from build123d import *

# Parameters (mm, degrees)
SCHIZZO1_W                               = 90
SCHIZZO1_H                               = 80
ESTRUSIONE_ESTRUSIONE1_DEPTH             = 10
RACCORDO1_R                              = 10
FORO_SVASATO_PER_VITE_M2_5_1_D           = 3.1
FORO_SVASATO_PER_VITE_M2_5_1_CSINK_D     = 5.5
FORO_SVASATO_PER_VITE_M2_5_1_CSINK_ANGLE = 90
SCHIZZO4_W                               = 30
SCHIZZO4_H                               = 15
ESTRUSIONE_ESTRUSIONE2_DEPTH             = 13
FORO_SVASATO_PER_VITE_M2_5_2_D           = 3.1
FORO_SVASATO_PER_VITE_M2_5_2_DEPTH       = 15
FORO_SVASATO_PER_VITE_M2_5_2_CSINK_D     = 5.5
FORO_SVASATO_PER_VITE_M2_5_2_CSINK_ANGLE = 90
FORO_SVASATO_PER_VITE_M2_5_2_TIP         = 0.931333959
RACCORDO2_R                              = 3
SCHIZZO5_R                               = 1.7
TAGLIO_ESTRUSIONE4_DEPTH                 = 15
TAGLIO_ESTRUSIONE5_START                 = -15
SCHIZZO6_R                               = 1.7
TAGLIO_ESTRUSIONE5_DEPTH                 = 15


with BuildPart() as part:
    # Schizzo1 → Estrusione-Estrusione1 (new body)
    with BuildSketch(Plane(origin=(0, 0, 0), x_dir=(1, 0, 0), z_dir=(0, 1, 0))):
        with Locations((-2.6, -4.4)):
            Rectangle(SCHIZZO1_W, SCHIZZO1_H)
    extrude(amount=ESTRUSIONE_ESTRUSIONE1_DEPTH)

    # Raccordo1
    raccordo1_edges = [part.edges().sort_by_distance(p)[0] for p in [
        (42.4, 5, -35.6),
        (42.4, 5, 44.4),
        (-47.6, 5, 44.4),
        (-47.6, 5, -35.6),
    ]]
    fillet(raccordo1_edges, radius=RACCORDO1_R)

    # Foro svasato per Vite M2.5-1 (through all)
    with Locations(Plane(origin=(12.4, 10, -15.6), x_dir=(0, 0, 1), z_dir=(0, 1, 0))):
        with Locations((0, 0), (40, 0)):
            CounterSinkHole(FORO_SVASATO_PER_VITE_M2_5_1_D / 2, FORO_SVASATO_PER_VITE_M2_5_1_CSINK_D / 2, counter_sink_angle=FORO_SVASATO_PER_VITE_M2_5_1_CSINK_ANGLE)

    # Schizzo4 → Estrusione-Estrusione2 (add)
    with BuildSketch(Plane(origin=(0, 10, 0), x_dir=(1, 0, 0), z_dir=(0, 1, 0))):
        with Locations((-17.6, 13.1)):
            Rectangle(SCHIZZO4_W, SCHIZZO4_H)
        with Locations((-17.6, -21.9)):
            Rectangle(SCHIZZO4_W, SCHIZZO4_H)
    extrude(amount=ESTRUSIONE_ESTRUSIONE2_DEPTH)

    # Foro svasato per Vite M2.5-2
    with Locations(Plane(origin=(-10.6, 14.5, 29.4), x_dir=(1, 0, 0), z_dir=(0, 0, 1))):
        with Locations((0, 0)):
            CounterSinkHole(FORO_SVASATO_PER_VITE_M2_5_2_D / 2, FORO_SVASATO_PER_VITE_M2_5_2_CSINK_D / 2, depth=FORO_SVASATO_PER_VITE_M2_5_2_DEPTH, counter_sink_angle=FORO_SVASATO_PER_VITE_M2_5_2_CSINK_ANGLE)
            with Locations((0, 0, -(FORO_SVASATO_PER_VITE_M2_5_2_DEPTH + FORO_SVASATO_PER_VITE_M2_5_2_TIP / 2))):  # 118° drill point
                Cone(0, FORO_SVASATO_PER_VITE_M2_5_2_D / 2, FORO_SVASATO_PER_VITE_M2_5_2_TIP, mode=Mode.SUBTRACT)

    # Raccordo2
    raccordo2_edges = [part.edges().sort_by_distance(p)[0] for p in [
        (-2.6, 16.5, -20.6),
        (-32.6, 16.5, -20.6),
        (-32.6, 16.5, -5.6),
        (-2.6, 16.5, -5.6),
        (-2.6, 16.5, 14.4),
        (-32.6, 16.5, 14.4),
        (-32.6, 16.5, 29.4),
        (-2.6, 16.5, 29.4),
    ]]
    fillet(raccordo2_edges, radius=RACCORDO2_R)

    # Schizzo5 → Taglio-Estrusione4 (cut)
    with BuildSketch(Plane(origin=(0, 0, -20.6), x_dir=(-1, 0, 0), z_dir=(0, 0, -1))):
        with Locations((10.6, 14.5)):
            Circle(SCHIZZO5_R)
        with Locations((24.6, 14.5)):
            Circle(SCHIZZO5_R)
    extrude(amount=-TAGLIO_ESTRUSIONE4_DEPTH, mode=Mode.SUBTRACT)

    # Schizzo6 → Taglio-Estrusione5 (cut)
    with BuildSketch(Plane.XY.offset(29.4).offset(TAGLIO_ESTRUSIONE5_START)):
        with Locations(Location((-24.6, 14.5, 0), (0, 0, 180))):
            Circle(SCHIZZO6_R)
    extrude(amount=TAGLIO_ESTRUSIONE5_DEPTH, mode=Mode.SUBTRACT)


solid = part.part
Geometry: final body of the model. Coordinates: model frame, mm. A direction names the side the tool comes from. Give positions to 0.01 mm unless a question says otherwise; leave off trailing zeros. Order: outer loops, then holes, each group sorted by start corner. A loop starts at its lowest first (then second) coordinate and runs counter-clockwise, first axis right, second up. Notation, with made-up numbers: (-18.5, 85.25) -> (34.5, 85.25) arc R18 ccw to (34.5, 108.25) -> close; hole circle Ø10 at (83.5, 24). An arc over 180 degrees is marked (long way). Answer as a JSON object with one key per item and string values.
Q1. Draft query along X for faces 5 (the cylindrical face through (-22.9, 14.43, 21.8)), 6 (the flat face through (-18, 16, -5.6)), 7 (the cylindrical face through (-3.46, 16.59, -6.5)). Return one class per face: released by +X, released by -X, zero draft, split by the parting line, or undercut.
Entries:
{"face 5": "undercut", "face 6": "zero draft", "face 7": "released by +X"}
Q2. Access query for faces 1 (the cylindrical face through (-31.74, 16.59, -19.7)), 2 (the flat face through (-2.6, 16, -13)), 3 (the flat face through (-18, 16, 29.4)), 4 (the flat face through (-18, 16, -20.6)). Directions: +Z, -Z, +X, -X, +Y, -Y. A direction counts if a zero-diameter tool reaches every point of the face in a straight line with its end or side. Return the directions, or none.
Entries:
{"face 1": "-Z, -X, +Y", "face 2": "+Z, -Z, +X, +Y", "face 3": "+Z, +X, -X, +Y", "face 4": "-Z, +X, -X, +Y"}
Q3. Material intervals for probe 1 along Y at (x, z) = (-24.6, 22); probe 2 along Z at (x, y) = (-28.5, 19); probe 3 along Z at (x, y) = (12.4, 7.25), sorted ascending.
Entries:
{"probe 1": "y = 0 to 12.8, 16.2 to 23", "probe 2": "z = -20.6 to -5.6, 14.4 to 29.4", "probe 3": "z = -35.6 to -17.15, -14.05 to 22.85, 25.95 to 44.4"}
Q4. Section D-D (y = 21.5). Output: boundary loops of the cut face in (x, z).
Entries:
{"outline": "(-32.6, -17.6) arc R3 ccw to (-29.6, -20.6) -> (-5.6, -20.6) arc R3 ccw to (-2.6, -17.6) -> (-2.6, -8.6) arc R3 ccw to (-5.6, -5.6) -> (-29.6, -5.6) arc R3 ccw to (-32.6, -8.6) -> close; (-32.6, 17.4) arc R3 ccw to (-29.6, 14.4) -> (-5.6, 14.4) arc R3 ccw to (-2.6, 17.4) -> (-2.6, 26.4) arc R3 ccw to (-5.6, 29.4) -> (-29.6, 29.4) arc R3 ccw to (-32.6, 26.4) -> close"}
Q5. Section B-B (y = 14.5). State how many separate pieces and enclosed holes the cut face has, plus the area to 3 significant figures.
Entries:
{"separate pieces": "6", "enclosed holes": "0", "area": "684 mm^2"}
Q6. Section C-C (x = 12.4). Output: boundary loops of the cut face in (y, z), plus the area to 3 significant figures.
Entries:
{"outline": "(0, -35.6) -> (10, -35.6) -> (10, -18.35) -> (8.8, -17.15) -> (0, -17.15) -> close; (0, -14.05) -> (8.8, -14.05) -> (10, -12.85) -> (10, 21.65) -> (8.8, 22.85) -> (0, 22.85) -> close; (0, 25.95) -> (8.8, 25.95) -> (10, 27.15) -> (10, 44.4) -> (0, 44.4) -> close", "area": "735 mm^2"}
Q7. First-contact query: pin 1 (10 mm diameter, centred on y = 18.5, z = 28, fed in from -X); pin 2 (5.5 mm diameter, centred on x = -24.6, y = 14.5, fed in from -Z); pin 3 (10.5 mm diameter, centred on x = -22.5, y = 19, fed in from +Z). Flat tips, straight axial feed; report the tip coordinate or a pass-through.
Entries:
{"pin 1": "stops at x = -32.6", "pin 2": "stops at z = -20.6", "pin 3": "stops at z = 29.4"}
Q8. Section A-A (z = 24.4). Output: boundary loops of the cut face in (x, y).
Entries:
{"outline": "(-47.6, 0) -> (10.85, 0) -> (10.85, 8.8) -> (9.65, 10) -> (-2.6, 10) -> (-2.6, 23) -> (-32.6, 23) -> (-32.6, 10) -> (-47.6, 10) -> close; (13.95, 0) -> (42.4, 0) -> (42.4, 10) -> (15.15, 10) -> (13.95, 8.8) -> close; hole circle Ø3.4 at (-24.6, 14.5); hole circle Ø3.1 at (-10.6, 14.5)"}
